Input: part model. Units: mm. Frame: model coordinates. A direction names the side the tool comes from. Give positions to 0.01 mm unless a question says otherwise; leave off trailing zeros. Loops run counter-clockwise (first coordinate to the right, second up) from the corner with the lowest first, then second, coordinate; pieces in that order, holes last. Notation, with made-up numbers: (0, 71.25) - (40, 71.25) arc R15 cw to (40, 82.25) - close; hole circle Ø11 at (-35.5, 51). An arc over 180 degrees is marked (long way). One line per item, written item: value.
from build123d import *

# Parameters (mm, degrees)
SKETCH1_W           = 85
SKETCH1_H           = 13
BOSS_EXTRUDE1_DEPTH = 5
SKETCH2_W           = 50
SKETCH2_H           = 3
CUT_EXTRUDE1_DEPTH  = 44.283946216
SKETCH3_W           = 5.833333
SKETCH3_H           = 5
SKETCH3_W_2         = 5.833334
SKETCH3_W_3         = 25
CUT_EXTRUDE2_DEPTH  = 44.283946216


with BuildPart() as part:
    # Sketch1 → Boss-Extrude1 (new body)
    with BuildSketch(Plane.XY):
        Rectangle(SKETCH1_W, SKETCH1_H)
    extrude(amount=BOSS_EXTRUDE1_DEPTH)

    # Sketch2 → Cut-Extrude1 (cut, through all)
    with BuildSketch(Plane.XY.offset(5)):
        Rectangle(SKETCH2_W, SKETCH2_H)
    extrude(amount=-CUT_EXTRUDE1_DEPTH, mode=Mode.SUBTRACT)

    # Sketch3 → Cut-Extrude2 (cut, through all)
    with BuildSketch(Plane(origin=(0, 0, 0), x_dir=(-1, 0, 0), z_dir=(0, 0, -1))):
        with Locations((-39.5833335, 4)):
            Rectangle(SKETCH3_W, SKETCH3_H)
        with Locations((-27.916667, 4)):
            Rectangle(SKETCH3_W_2, SKETCH3_H)
        with Locations((-12.5, 4)):
            Rectangle(SKETCH3_W_3, SKETCH3_H)
        with Locations((12.5, 4)):
            Rectangle(SKETCH3_W_3, SKETCH3_H)
        with Locations((27.916667, 4)):
            Rectangle(SKETCH3_W_2, SKETCH3_H)
        with Locations((39.5833335, 4)):
            Rectangle(SKETCH3_W, SKETCH3_H)
    extrude(amount=-CUT_EXTRUDE2_DEPTH, mode=Mode.SUBTRACT)


solid = part.part
Item 1: Material intervals for L1, parallel to X at y = 5.5, z = 4.15; L2, parallel to X at y = 0.25, z = 3.45; L3, parallel to Y at x = 3, z = 2.7, sorted ascending.
Verdict:
L1: x = -36.67 to -30.83, 30.83 to 36.67
L2: x = -42.5 to -25, 25 to 42.5
L3: y = -6.5 to -1.5
Item 2: Section B-B, the plane z = 1.75. Output: boundary loops of the cut face in (x, y).
Verdict:
outline: (-42.5, -6.5) - (42.5, -6.5) - (42.5, 1.5) - (36.67, 1.5) - (36.67, 6.5) - (30.83, 6.5) - (30.83, 1.5) - (25, 1.5) - (25, -1.5) - (-25, -1.5) - (-25, 1.5) - (-30.83, 1.5) - (-30.83, 6.5) - (-36.67, 6.5) - (-36.67, 1.5) - (-42.5, 1.5) - close
Item 3: Section C-C, the plane x = 5. Output: boundary loops of the cut face in (y, z).
Verdict:
outline: (-6.5, 0) - (-1.5, 0) - (-1.5, 5) - (-6.5, 5) - close
Item 4: Draft query along X for faces 1 (the face through (-36.667, 4, 2)), 2 (the face through (-25, 0, 3)), 3 (the face through (0, -1.5, 3)), 4 (the face through (-40, 1.5, 2)). Return one class per face: pulls with the +X half, pulls with the -X half, needs draft (parallel to the pull), parting line crosses it, or undercut.
Verdict:
face 1: pulls with the -X half
face 2: undercut
face 3: undercut
face 4: needs draft
Item 5: Access query for faces 5 (the face through (25, 0, 3)), 6 (the face through (40, 1.5, 2)), 7 (the face through (42.5, -3, 2)). Directions: +Z, -Z, +X, -X, +Y, -Y. A direction counts if a zero-diameter tool reaches every point of the face in a straight line with its end or side. Return the directions, or none.
Verdict:
face 5: +Z, -Z, +Y
face 6: +Z, -Z, +X, +Y
face 7: +Z, -Z, +X, +Y, -Y
Item 6: Section D-D, the plane y = 5.5. Output: boundary loops of the cut face in (x, z), and give its area (3 significant figures).
Verdict:
outline: (-36.67, 0) - (-30.83, 0) - (-30.83, 5) - (-36.67, 5) - close; (30.83, 0) - (36.67, 0) - (36.67, 5) - (30.83, 5) - close
area: 58.3 mm^2
Item 7: Pin query (flat end, axial travel): P1, Ø2.5, axis at x = 38, z = 3, coming from the +Y side; P2, Ø2.5, axis at y = 3, z = 3, coming from the -X side. Return the tip coordinate at first contact, or that it passes through.
Verdict:
P1: stops at y = 1.5
P2: stops at x = -36.67
Item 8: Section A-A, the plane y = -0.75. Output: boundary loops of the cut face in (x, z).
Verdict:
outline: (-42.5, 0) - (-25, 0) - (-25, 5) - (-42.5, 5) - close; (25, 0) - (42.5, 0) - (42.5, 5) - (25, 5) - close
